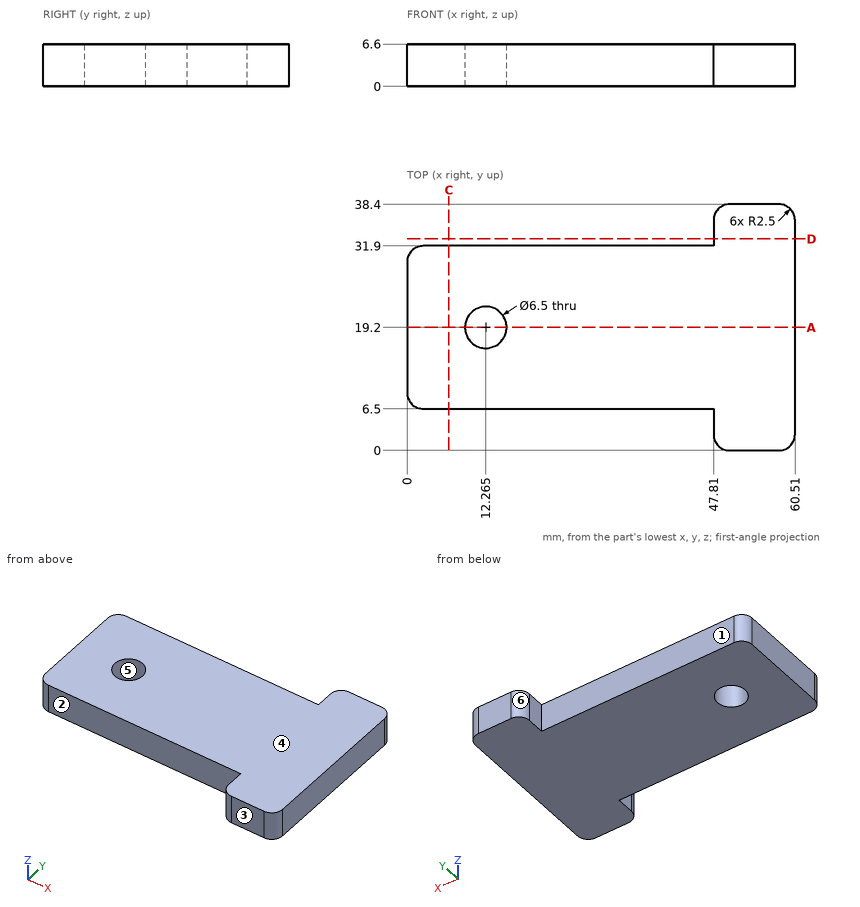
Geometry: see drawing. Coordinates: mm, zero at the bounding-box minimum. A direction names the side the tool comes from. Round coordinates to 2 decimals unless told otherwise and drop trailing zeros. Loops run counter-clockwise (first coordinate to the right, second up) from the corner with the lowest first, then second, coordinate; pieces in that order, holes last.
(1) Section query C-C (x = 6.5). Output: boundary loops of the cut face in (y, z), and give its area (3 significant figures).
From the geometry:
outline: (6.5, 0) - (31.9, 0) - (31.9, 6.6) - (6.5, 6.6) - close
area: 168 mm2
(2) Pull-direction query (Y, two-part tool) for the marked faces 4, 5 and 6; classes: +Y half, -Y half, draft (parallel to the pull), parting line (faces both ways), or undercut.
From the geometry:
face 4: draft
face 5: undercut
face 6: +Y half
(3) Section query D-D (y = 33). Output: boundary loops of the cut face in (x, z), and give its area (3 significant figures).
From the geometry:
outline: (47.81, 0) - (60.51, 0) - (60.51, 6.6) - (47.81, 6.6) - close
area: 83.8 mm2
(4) Material intervals for probe 1 along Y at (x, z) = (20, 5.5); probe 2 along Y at (x, z) = (11.5, 2.25); probe 3 along X at (y, z) = (29.5, 1), sorted ascending.
From the geometry:
probe 1: y = 6.5 to 31.9
probe 2: y = 6.5 to 16.04, 22.36 to 31.9
probe 3: x = 0 to 60.51
(5) Section query A-A (y = 19.2). Output: boundary loops of the cut face in (x, z) (1 decimal).
From the geometry:
outline: (0, 0) - (9, 0) - (9, 6.6) - (0, 6.6) - close; (15.5, 0) - (60.5, 0) - (60.5, 6.6) - (15.5, 6.6) - close
(6) Access query for the marked faces 1, 2 and 3. Directions: +Z, -Z, +X, -X, +Y, -Y. A direction counts if a zero-diameter tool reaches every point of the face in a straight line with its end or side. Return the directions, or none.
From the geometry:
face 1: +Z, -Z, -X, +Y
face 2: +Z, -Z, -X, -Y
face 3: +Z, -Z, +X, -X, -Y
(7) Contact query for flat-ended pins moving along their axis: pin 1 Ø3.5 at (x, z) = (17, 2.5) entering from -Y; pin 2 Ø1 at (x, z) = (46, 2) entering from +Y; pin 3 Ø2 at (y, z) = (4, 4.5) entering from -X; pin 4 Ø5 at (x, y) = (12.26, 19.2) entering from +Z. Output: stop coordinate, or through.
From the geometry:
pin 1: stops at y = 6.5
pin 2: stops at y = 31.9
pin 3: stops at x = 47.81
pin 4: passes through
